Model file for the job. Use its own axes, mm. A direction names the side the tool comes from. Round coordinates to 2 decimals unless told otherwise and drop trailing zeros. Loops run counter-clockwise (first coordinate to the right, second up) from the corner with the lowest first, then second, coordinate; pieces in that order, holes last. Notation, with made-up numbers: M 3,21.25 L 43,21.25 A17 cw 43,40.25 Z; hole C 14,-1.5 d11. An arc over 180 degrees is marked long. Answer in a Markdown table with one row per item.
from build123d import *

# Parameters (mm, degrees)
CROQUIS1_W              = 26
CROQUIS1_H              = 26
SALIENTE_EXTRUIR1_DEPTH = 1
CROQUIS2_R              = 10.5
SALIENTE_EXTRUIR2_DEPTH = 44.5
SALIENTE_EXTRUIR3_DEPTH = 1
CROQUIS4_R              = 6
CORTAR_EXTRUIR1_DEPTH   = 51.13481824


with BuildPart() as part:
    # Croquis1 → Saliente-Extruir1 (new body)
    with BuildSketch(Plane.XY):
        Rectangle(CROQUIS1_W, CROQUIS1_H)
    extrude(amount=SALIENTE_EXTRUIR1_DEPTH)

    # Croquis2 → Saliente-Extruir2 (add)
    with BuildSketch(Plane.XY.offset(1)):
        Circle(CROQUIS2_R)
    extrude(amount=SALIENTE_EXTRUIR2_DEPTH)

    # Croquis3 → Saliente-Extruir3 (add)
    with BuildSketch(Plane.XY.offset(45.5)):
        with BuildLine():
            ThreePointArc((10.5, 0), (0, -10.5), (-10.5, 0))
            Line((-10.5, 0), (-13.5, 0))
            Line((-13.5, 0), (-13.5, -5))
            Line((-13.5, -5), (-8.766919396, -8.910169713))
            ThreePointArc((-8.766919396, -8.910169713), (0, -12.063114964), (8.766919396, -8.910169713))
            Line((8.766919396, -8.910169713), (13.5, -5))
            Line((13.5, -5), (13.5, 0))
            Line((13.5, 0), (10.5, 0))
        make_face()
        with BuildLine():
            Line((-13.5, 0), (-10.5, 0))
            ThreePointArc((-10.5, 0), (0, 10.5), (10.5, 0))
            Line((10.5, 0), (13.5, 0))
            Line((13.5, 0), (13.5, 5))
            Line((13.5, 5), (8.766919396, 8.910169713))
            ThreePointArc((8.766919396, 8.910169713), (0, 12.063114964), (-8.766919396, 8.910169713))
            Line((-8.766919396, 8.910169713), (-13.5, 5))
            Line((-13.5, 5), (-13.5, 0))
        make_face()
        with BuildLine():
            Line((10.5, 0), (0, 0))
            Line((0, 0), (-10.5, 0))
            ThreePointArc((-10.5, 0), (0, -10.5), (10.5, 0))
        make_face()
        with BuildLine():
            Line((-10.5, 0), (0, 0))
            Line((0, 0), (10.5, 0))
            ThreePointArc((10.5, 0), (0, 10.5), (-10.5, 0))
        make_face()
    extrude(amount=SALIENTE_EXTRUIR3_DEPTH)

    # Croquis4 → Cortar-Extruir1 (cut, through all)
    with BuildSketch(Plane.XY.offset(46.5)):
        Circle(CROQUIS4_R)
    extrude(amount=-CORTAR_EXTRUIR1_DEPTH, mode=Mode.SUBTRACT)


solid = part.part
1. Mould opens along Y. For faces 1 (the cylindrical face through (-0.133, -12.062, 45.993)), 2 (the flat face through (-11.1, 6.982, 45.993)), 3 (the cylindrical face through (-6, 0, 24)), 4 (the flat face through (-13.5, 0, 46)) say: +Y half, -Y half, draft (parallel to the pull), parting line (faces both ways), or undercut.
Verdict:
| item | result |
|---|---|
| face 1 | -Y half |
| face 2 | +Y half |
| face 3 | undercut |
| face 4 | draft |
2. Wall check: probe 1 along Y at (x, z) = (0, 13); probe 2 along Z at (x, y) = (12.25, -4.5); probe 3 along X at (y, z) = (0.25, 40). Give the ranges that are in metal, low to high.
Verdict:
| item | result |
|---|---|
| probe 1 | y = -10.5 to -6, 6 to 10.5 |
| probe 2 | z = 0 to 1, 45.5 to 46.5 |
| probe 3 | x = -10.5 to -5.99, 5.99 to 10.5 |
3. Pin check, flat tips, straight feed: pin 1 (2 mm diameter, centred on y = -2, z = 18, fed in from +X); pin 2 (4 mm diameter, centred on y = 4.5, z = 5, fed in from -X); pin 3 (2 mm diameter, centred on y = -5.5, z = 40, fed in from -X); pin 4 (1.5 mm diameter, centred on x = 0.5, y = 4.5, fed in from +Z). Stop position of each tip, or through.
Verdict:
| item | result |
|---|---|
| pin 1 | stops at x = 10.45 |
| pin 2 | stops at x = -10.2 |
| pin 3 | stops at x = -9.49 |
| pin 4 | passes through |
4. Saw through at A-A (y = 0). Write the cut outline in (x, z), and give its area (4 significant figures).
Verdict:
| item | result |
|---|---|
| outline | M -13.5,45.5 L -10.5,45.5 L -10.5,1 L -13,1 L -13,0 L -6,0 L -6,46.5 L -13.5,46.5 Z; M 6,0 L 13,0 L 13,1 L 10.5,1 L 10.5,45.5 L 13.5,45.5 L 13.5,46.5 L 6,46.5 Z |
| area | 429.5 mm² |
5. Saw through at C-C (z = 40). Write the cut outline in (x, y), and give its area (3 significant figures).
Verdict:
| item | result |
|---|---|
| outline | C 0,0 d21; hole C 0,0 d12 |
| area | 233 mm² |
6. Saw through at D-D (y = 7). Write the cut outline in (x, z), and give its area (3 significant figures).
Verdict:
| item | result |
|---|---|
| outline | M -13,0 L 13,0 L 13,1 L 7.83,1 L 7.83,45.5 L 11.08,45.5 L 11.08,46.5 L -11.08,46.5 L -11.08,45.5 L -7.83,45.5 L -7.83,1 L -13,1 Z |
| area | 745 mm² |
7. Saw through at B-B (x = 0). Write the cut outline in (y, z), and give its area (3 significant figures).
Verdict:
| item | result |
|---|---|
| outline | M -13,0 L -6,0 L -6,46.5 L -12.06,46.5 L -12.06,45.5 L -10.5,45.5 L -10.5,1 L -13,1 Z; M 6,0 L 13,0 L 13,1 L 10.5,1 L 10.5,45.5 L 12.06,45.5 L 12.06,46.5 L 6,46.5 Z |
| area | 427 mm² |
8. Tool access for faces 5 (the flat face through (4, 10, 45.5)), 6 (the flat face through (11.1, -6.982, 45.993)), 7 (the flat face through (11.2, 6.9, 46)): list every direction of +Z, -Z, +X, -X, +Y, -Y with a clear straight run to the whole face (end or side of a thin tool).
Verdict:
| item | result |
|---|---|
| face 5 | none |
| face 6 | +Z, +X, -Y |
| face 7 | +Z, +X, +Y |
